Check sheet for the modelled part. Datum: model origin and axes. Units: mm. A direction names the side the tool comes from. Round coordinates to 2 decimals unless told otherwise and drop trailing zeros. Write each loop counter-clockwise with the first axis right and the second up, starting at its lowest first coordinate (ties: lowest second). Pieces come first, ordered by that corner, then holes. Notation, with made-up numbers: (-21.5, 67.25) -> (22.5, 67.25) arc R9 ccw to (22.5, 74.25) -> close; hole circle Ø5 at (12.25, 29). An arc over 180 degrees is marked (long way). Answer as a JSON object with one key per item and string values. Group by question number.
```python
from build123d import *

# Parameters (mm, degrees)
BOSS_EXTRUDE1_DEPTH = 38.1
SKETCH2_R           = 1.5875
CUT_EXTRUDE1_DEPTH  = 45.45
SKETCH3_R           = 1.5875
CUT_EXTRUDE2_DEPTH  = 45.45


with BuildPart() as part:
    # Sketch1 → Boss-Extrude1 (new body)
    with BuildSketch(Plane.XY):
        Polygon((0, 12.7), (0, 0), (19.05, 0), (19.05, 1.5875), (1.5875, 1.5875), (1.5875, 12.7), align=None)
    extrude(amount=BOSS_EXTRUDE1_DEPTH)

    # Sketch2 → Cut-Extrude1 (cut, through all)
    with BuildSketch(Plane.ZY):
        with Locations(Location((19.05, 6.35, 0), (0, 0, 270))):
            Circle(SKETCH2_R)
    extrude(amount=-CUT_EXTRUDE1_DEPTH, mode=Mode.SUBTRACT)

    # Sketch3 → Cut-Extrude2 (cut, through all)
    with BuildSketch(Plane.XZ):
        with Locations(Location((6.35, 4.1275, 0), (0, 0, 270))):
            Circle(SKETCH3_R)
        with Locations(Location((6.35, 33.9725, 0), (0, 0, 270))):
            Circle(SKETCH3_R)
    extrude(amount=-CUT_EXTRUDE2_DEPTH, mode=Mode.SUBTRACT)


solid = part.part
```
(1) Section check A-A on x = 6.35. Record the cut outline in (y, z) (1 decimal).
(2) Access from +Z, -Z, +X, -X, +Y, -Y to the whole of each face (thin tool, end or side, straight path). Record for faces 1 (the flat face through (10, 1.588, 19)), 2 (the flat face through (1, 12.7, 19)).
(3) Section check B-B on z = 19.05. Record the cut outline in (x, y).
(4) Scan lines: line 1 along Z through (x, y) = (7.75, 1.5); line 2 along X through (y, z) = (12, 32.5). Record each from-to range of solid material in increasing order.
(5) Section check D-D on z = 29.5. Record the cut outline in (x, y).
(6) Section check C-C on y = 6.35. Record the cut outline in (x, z), then the cut area to 3 significant figures.
(7) Release check for a two-part mould opening along Z. For faces 3 (the flat face through (6, 1, 0)), 4 (the flat face through (9, 0, 19)), 5 (the cylindrical face through (5.38, 0.78, 35.23)) record: pulls with the +Z half, pulls with the -Z half, needs draft (parallel to the pull), parting line crosses it, or undercut.
(8) Go/stop test with flat-tipped pins: pin 1 Ø3.5 at (y, z) = (6.35, 19.05) entering from -X; pin 2 Ø5 at (x, z) = (8, 18.5) entering from +Y. Record where each tip stops, or that it passes through.
Data:
{
 "1": {"outline": "(0, 0) -> (1.6, 0) -> (1.6, 2.5) -> (0, 2.5) -> close; (0, 5.7) -> (1.6, 5.7) -> (1.6, 32.4) -> (0, 32.4) -> close; (0, 35.6) -> (1.6, 35.6) -> (1.6, 38.1) -> (0, 38.1) -> close"},
 "2": {"face 1": "+Z, -Z, +X, +Y", "face 2": "+Z, -Z, +X, -X, +Y"},
 "3": {"outline": "(0, 0) -> (19.05, 0) -> (19.05, 1.59) -> (1.59, 1.59) -> (1.59, 4.76) -> (0, 4.76) -> close; (0, 7.94) -> (1.59, 7.94) -> (1.59, 12.7) -> (0, 12.7) -> close"},
 "4": {"line 1": "z = 0 to 3.38, 4.88 to 33.22, 34.72 to 38.1", "line 2": "x = 0 to 1.59"},
 "5": {"outline": "(0, 0) -> (19.05, 0) -> (19.05, 1.59) -> (1.59, 1.59) -> (1.59, 12.7) -> (0, 12.7) -> close"},
 "6": {"outline": "(0, 0) -> (1.59, 0) -> (1.59, 17.46) -> (0, 17.46) -> close; (0, 20.64) -> (1.59, 20.64) -> (1.59, 38.1) -> (0, 38.1) -> close", "area": "55.4 mm²"},
 "7": {"face 3": "pulls with the -Z half", "face 4": "needs draft", "face 5": "undercut"},
 "8": {"pin 1": "stops at x = 0", "pin 2": "stops at y = 1.59"}
}
